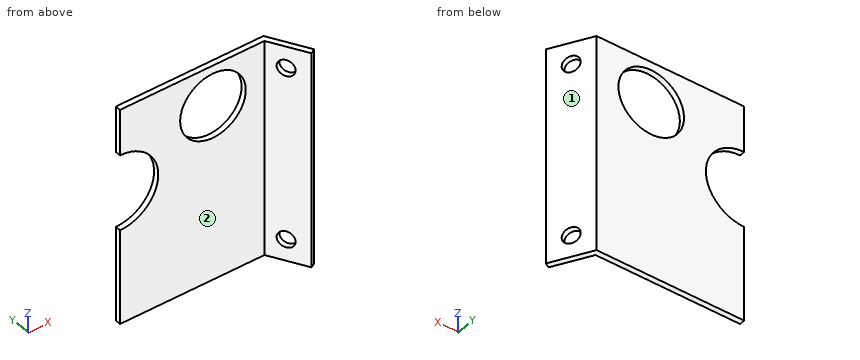
```python
from build123d import *

# Parameters (mm, degrees)
BOSS_EXTRUDE1_DEPTH = 40
SKETCH2_R           = 1.5
CUT_EXTRUDE1_DEPTH  = 40
SKETCH3_R           = 7
SKETCH3_R_2         = 6
CUT_EXTRUDE2_DEPTH  = 40


with BuildPart() as part:
    # Sketch1 → Boss-Extrude1 (new body)
    with BuildSketch(Plane.XY):
        Polygon((0, 0), (27, 0), (31, -6.92820323), (30.133974596, -7.42820323), (26.422649731, -1), (0, -1), align=None)
    extrude(amount=BOSS_EXTRUDE1_DEPTH)

    # Sketch2 → Cut-Extrude1 (cut)
    with BuildSketch(Plane(origin=(20.25, 11.691342951, 0), x_dir=(0, 0, -1), z_dir=(0.86602540378444, 0.4999999999999978, 0))):
        with Locations(Location((-36, -17.5, 0), (0, 0, 90))):
            Circle(SKETCH2_R)
        with Locations(Location((-4, -17.5, 0), (0, 0, 90))):
            Circle(SKETCH2_R)
    extrude(amount=-CUT_EXTRUDE1_DEPTH, mode=Mode.SUBTRACT)

    # Sketch3 → Cut-Extrude2 (cut)
    with BuildSketch(Plane(origin=(0, 0, 0), x_dir=(-1, 0, 0), z_dir=(0, 1, 0))):
        with Locations((0, 24.5)):
            Circle(SKETCH3_R)
        with Locations(Location((-17, 32.5, 0), (0, 0, 90))):
            Circle(SKETCH3_R_2)
    extrude(amount=-CUT_EXTRUDE2_DEPTH, mode=Mode.SUBTRACT)


solid = part.part
```
The listing builds one solid part. Answer for the finished solid, in the listing's coordinates (mm). Face numbers are marked on the shaded views. A direction names the side the tool comes from. Coordinates: 2 decimals unless noted, no trailing zeros. Order: outer loops, then holes, each group sorted by start corner. A loop starts at its lowest first (then second) coordinate and runs counter-clockwise, first axis right, second up. Notation, with made-up numbers: M 57.25,84 L 67.25,84 A22 ccw 67.25,92 Z; hole C 80.5,68.25 d3. An arc over 180 degrees is marked long. Answer as a JSON object with one key per item and string values. Group by question number.
1. A tool of negligible diameter and unlimited length cuts with its end or side. For the marked faces 1 and 2, from which of +Z, -Z, +X, -X, +Y, -Y can it reach the whole face along a straight path? Write none if from no direction.
2. Straight lines are drawn through the part: line 1 (X direction, y = -0.65, z = 32.5); line 2 (Y direction, x = 26, z = 32); line 3 (X direction, y = -0.4, z = 32.5). For each, find the intervals that lie inside material, in ascending order.
3. Section A-A on x = 17 is taken. Write down the section's boundary in (y, z), then the cut area to 3 significant figures.
4. Section D-D on z = 24.5 is taken. Write down the section's boundary in (x, y).
5. Section B-B on z = 37 is taken. Write down the section's boundary in (x, y), then the cut area to 3 significant figures.
6. Flat-ended cylindrical pins translate along their axes: P1, Ø1, axis at x = 5.5, z = 5.5, coming from the -Y side; P2, Ø12, axis at x = 11.5, z = 17.5, coming from the +Y side; P3, Ø2, axis at y = -6, z = 25.5, coming from the +X side. Find the tip coordinate at first contact, or state that the pin passes through.
7. Section C-C on y = -0.5 is taken. Write down the section's boundary in (x, z), then the cut area to 3 significant figures.
Values follow:
{
 "1": {"face 1": "+Z, -Z, +X, +Y", "face 2": "+Z, -Z, -X, -Y"},
 "2": {"line 1": "0 to 11, 23 to 27.38", "line 2": "-1 to 0", "line 3": "0 to 11, 23 to 27.23"},
 "3": {"outline": "M -1,0 L 0,0 L 0,26.5 L -1,26.5 Z; M -1,38.5 L 0,38.5 L 0,40 L -1,40 Z", "area": "28.0 mm2"},
 "4": {"outline": "M 7,-1 L 26.42,-1 L 30.13,-7.43 L 31,-6.93 L 27,0 L 7,0 Z"},
 "5": {"outline": "M 0,-1 L 13.03,-1 L 13.03,0 L 0,0 Z; M 20.97,-1 L 26.42,-1 L 27.57,-3 L 28.44,-2.5 L 27,0 L 20.97,0 Z; M 28.69,-4.93 L 30.13,-7.43 L 31,-6.93 L 29.56,-4.43 Z", "area": "24.2 mm2"},
 "6": {"P1": "y = -1", "P2": "y = 0", "P3": "x = 31"},
 "7": {"outline": "M 0,0 L 27.29,0 L 27.29,40 L 0,40 L 0,31.5 A7 cw 0,17.5 Z; hole C 17,32.5 d12", "area": "901 mm2"}
}
